Read the model definition and answer for the solid it produces. Units are mm, in the model's axes. A direction names the side the tool comes from. Give positions to 0.01 mm unless a question says otherwise; leave off trailing zeros. Loops run counter-clockwise (first coordinate to the right, second up) from the corner with the lowest first, then second, coordinate; pieces in that order, holes last. Notation, with made-up numbers: (82, -36) -> (95, -36) arc R15 cw to (95, -21) -> close; hole circle Ø4 at (25, 42.25). An arc over 180 degrees is marked (long way). Return JSON: item names as keys, results as strings. Group by question number.
from build123d import *

# Parameters (mm, degrees)
F1_DEPTH     = 100
F2_T1_DEPTH  = 105.8849898869
F2_T3_DEPTH  = 114.5074829388
F2_T5_DEPTH  = 114.0858604347
F2_T7_DEPTH  = 114.5074829388
F2_T9_DEPTH  = 114.0858604347
F2_T12_ANGLE = 196
F2_T14_ANGLE = 196
F2_T16_ANGLE = 196
F2_T18_ANGLE = 196


# Not quite as in the source:
# - a fillet or chamfer that OpenCascade refuses, or shapes differently, is made with other operations: its cross-section is extruded or revolved along the edge and cut away or added


with BuildPart() as f1:
    # F0 (on Front) → F1 (new body)
    with BuildSketch(Plane.XZ):
        with BuildLine():
            Line((-61.9215476124, -110.8464484404), (-77.5, 0))
            ThreePointArc((-77.5, 0), (0, 89.1535515596), (77.5, 0))
            Line((77.5, 0), (61.9215476124, -110.8464484404))
            Line((61.9215476124, -110.8464484404), (64.95103033, -110.8464484404))
            Line((64.95103033, -110.8464484404), (80.4708042062, -0.4175193029))
            ThreePointArc((80.4708042062, -0.4175193029), (0, 92.1535515596), (-80.4708042062, -0.4175193029))
            Line((-80.4708042062, -0.4175193029), (-64.95103033, -110.8464484404))
            Line((-64.95103033, -110.8464484404), (-61.9215476124, -110.8464484404))
        make_face()
    extrude(amount=F1_DEPTH)

    # F2: chamfer of 1 on 17 edges, made by hand

    # F2_s2 → F2_t1 (cut)
    with BuildSketch(Plane.XZ.offset(-2.9424949434)):
        Polygon((-63.0719160196, -110.8464484404), (-62.0816479509, -109.7072753394), (-61.9215476124, -110.8464484404), align=None)
    extrude(amount=F2_T1_DEPTH, mode=Mode.SUBTRACT)

    # F2_s4 → F2_t3 (cut)
    with BuildSketch(Plane(origin=(14.4352522013, 0, -102.7121564484), x_dir=(0, 1, 0), z_dir=(-0.139173101, 0, 0.9902680687))):
        Polygon((-1, 76.7457753275), (0, 77.7457753275), (0, 76.7457753275), align=None)
        Polygon((-99, 76.7457753275), (-100, 77.7457753275), (-100, 76.7457753275), align=None)
    extrude(amount=F2_T3_DEPTH, mode=Mode.SUBTRACT)

    # F2_s6 → F2_t5 (cut)
    with BuildSketch(Plane(origin=(-1.5011092824, 0, 10.6809475379), x_dir=(0, 1, 0), z_dir=(0.139173101, 0, -0.9902680687))):
        Polygon((-1, -79.7457753275), (0, -78.7457753275), (0, -79.7457753275), align=None)
        Polygon((-99, -79.7457753275), (-100, -78.7457753275), (-100, -79.7457753275), align=None)
    extrude(amount=F2_T5_DEPTH, mode=Mode.SUBTRACT)

    # F2_s8 → F2_t7 (cut)
    with BuildSketch(Plane(origin=(1.5011092824, 0, 10.6809475379), x_dir=(0, 1, 0), z_dir=(-0.139173101, 0, -0.9902680687))):
        Polygon((-1, 76.7457753275), (0, 77.7457753275), (0, 76.7457753275), align=None)
        Polygon((-99, 76.7457753275), (-100, 77.7457753275), (-100, 76.7457753275), align=None)
    extrude(amount=F2_T7_DEPTH, mode=Mode.SUBTRACT)

    # F2_s10 → F2_t9 (cut)
    with BuildSketch(Plane(origin=(-14.37657369, 0, -102.2946371455), x_dir=(0, 1, 0), z_dir=(0.139173101, 0, 0.9902680687))):
        Polygon((-1, -79.7457753275), (0, -78.7457753275), (0, -79.7457753275), align=None)
        Polygon((-99, -79.7457753275), (-100, -78.7457753275), (-100, -79.7457753275), align=None)
    extrude(amount=F2_T9_DEPTH, mode=Mode.SUBTRACT)

    # F2_s11 → F2_t12 (revolve, cut)
    with BuildSketch(Plane(origin=(1.5011092824, 0, 10.6809475379), x_dir=(0, 1, 0), z_dir=(-0.139173101, 0, -0.9902680687))):
        Polygon((-1, 79.7457753275), (0, 78.7457753275), (0, 79.7457753275), align=None)
    revolve(axis=Axis((0, 0, 10.8919146894), (0, -1, 0)), revolution_arc=F2_T12_ANGLE, mode=Mode.SUBTRACT)

    # F2_s13 → F2_t14 (revolve, cut)
    with BuildSketch(Plane(origin=(1.5011092824, 0, 10.6809475379), x_dir=(0, 1, 0), z_dir=(-0.139173101, 0, -0.9902680687))):
        Polygon((-99, 79.7457753275), (-100, 78.7457753275), (-100, 79.7457753275), align=None)
    revolve(axis=Axis((0, -100, 10.8919146894), (0, -1, 0)), revolution_arc=F2_T14_ANGLE, mode=Mode.SUBTRACT)

    # F2_s15 → F2_t16 (revolve, cut)
    with BuildSketch(Plane(origin=(-1.5011092824, 0, 10.6809475379), x_dir=(0, 1, 0), z_dir=(0.139173101, 0, -0.9902680687))):
        Polygon((-1, -76.7457753275), (0, -77.7457753275), (0, -76.7457753275), align=None)
    revolve(axis=Axis((0, 0, 10.8919146894), (0, 1, 0)), revolution_arc=F2_T16_ANGLE, mode=Mode.SUBTRACT)

    # F2_s17 → F2_t18 (revolve, cut)
    with BuildSketch(Plane(origin=(-1.5011092824, 0, 10.6809475379), x_dir=(0, 1, 0), z_dir=(0.139173101, 0, -0.9902680687))):
        Polygon((-99, -76.7457753275), (-100, -77.7457753275), (-100, -76.7457753275), align=None)
    revolve(axis=Axis((0, -100, 10.8919146894), (0, 1, 0)), revolution_arc=F2_T18_ANGLE, mode=Mode.SUBTRACT)


solid = f1.part
1. Section B-B on z = -43 is taken. Determine the outline of the cut face in (x, y), then the cut area to 3 significant figures.
2. Flat-ended cylindrical pins translate along their axes: pin 1 Ø10 at (y, z) = (-56.5, 10) entering from +X; pin 2 Ø5 at (y, z) = (-17, 59) entering from -X; pin 3 Ø5 at (y, z) = (-73.5, -7.5) entering from +X; pin 4 Ø10 at (x, y) = (-62.5, -74) entering from -Z. Find the tip coordinate at first contact, or state that the pin passes through.
3. Section C-C on x = 0 is taken. Determine the outline of the cut face in (y, z), then the cut area to 3 significant figures.
4. Determine the mould class of faces 1 (the conical face through (-1.88, -0.83, 89.3)), 2 (the flat face through (72.1, -0.5, -56.4)) for opening direction Z: pulls with the +Z half, pulls with the -Z half, needs draft (parallel to the pull), parting line crosses it, or undercut.
5. Straight lines are drawn through the part: line 1 (Z direction, x = 0, y = -78); line 2 (X direction, y = -16, z = 27.5); line 3 (X direction, y = -26.5, z = -90). For each, find the intervals that lie inside material, in ascending order. Write a range as from..to.
6. Section A-A on y = -26.5 is taken. Determine the outline of the cut face in (x, z).
7. Which of the six approach directions +Z, -Z, +X, -X, +Y, -Y give full straight-line access (tool end or side, diameter ignored) to faces 3 (the flat face through (69.82, -49.31, -54.65)), 4 (the flat face through (-70.11, -99.493, -56.127)), 5 (the flat face through (-72.82, -49.31, -54.86)), 6 (the flat face through (72.602, -49.314, -56.405)), 7 (the flat face through (70.308, -0.507, -54.716))?
Completed:
{
 "1": {"outline": "(-74.49, -99) -> (-73.48, -100) -> (-72.47, -100) -> (-71.46, -99) -> (-71.46, -1) -> (-72.47, 0) -> (-73.48, 0) -> (-74.49, -1) -> close; (71.46, -99) -> (72.47, -100) -> (73.48, -100) -> (74.49, -99) -> (74.49, -1) -> (73.48, 0) -> (72.47, 0) -> (71.46, -1) -> close", "area": "602 mm²"},
 "2": {"pin 1": "stops at x = 81.26", "pin 2": "stops at x = -67.26", "pin 3": "stops at x = 79.83", "pin 4": "stops at z = -110.85"},
 "3": {"outline": "(-100, 90.15) -> (-99, 89.15) -> (-1, 89.15) -> (0, 90.15) -> (0, 91.15) -> (-1, 92.15) -> (-99, 92.15) -> (-100, 91.15) -> close", "area": "298 mm²"},
 "4": {"face 1": "undercut", "face 2": "pulls with the -Z half"},
 "5": {"line 1": "z = 89.15..92.15", "line 2": "x = -79.55..-76.48, 76.48..79.55", "line 3": "x = -67.88..-64.85, 64.85..67.88"},
 "6": {"outline": "(-80.47, -0.42) -> (-64.95, -110.85) -> (-63.07, -110.85) -> (-62.08, -109.71) -> (-77.5, 0) arc R78.26 cw (long way) to (77.5, 0) -> (61.92, -110.85) -> (64.95, -110.85) -> (80.47, -0.42) arc R81.26 ccw (long way) to start"},
 "7": {"face 3": "+Y, -Y", "face 4": "-Y", "face 5": "-Z, -X, +Y, -Y", "face 6": "-Z, +X, +Y, -Y", "face 7": "+Y"}
}
